Design review of the part built by this model. Coordinates are the model's own, in mm. Face numbers are marked on the shaded views. A direction names the side the tool comes from. Give positions to 0.01 mm unless a question says otherwise; leave off trailing zeros. Order: outer loops, then holes, each group sorted by start corner. A loop starts at its lowest first (then second) coordinate and runs counter-clockwise, first axis right, second up.
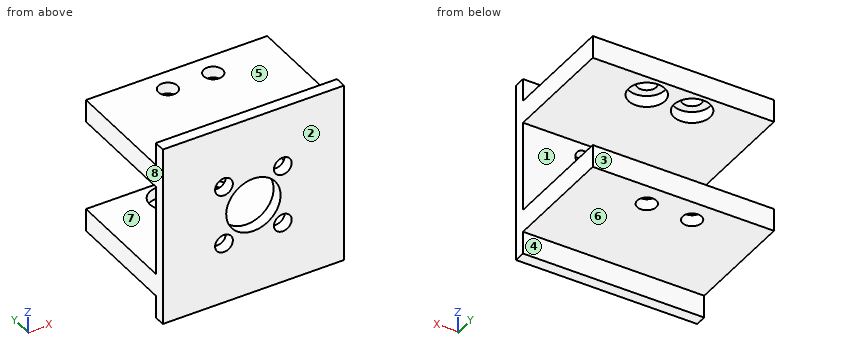
```python
from build123d import *

# Parameters (mm, degrees)
SKETCH1_W           = 50.8
SKETCH1_H           = 50.8
SKETCH1_R           = 2.4892
SKETCH1_R_2         = 7.62
BOSS_EXTRUDE1_DEPTH = 3.175
SKETCH2_W           = 50.8
SKETCH2_H           = 6.35
BOSS_EXTRUDE2_DEPTH = 31.75
CUT_EXTRUDE1_REACH  = 63.974
SKETCH3_R           = 2.667
SKETCH5_R           = 5.08
CUT_EXTRUDE2_DEPTH  = 3.175
CUT_EXTRUDE3_START  = -3.175
SKETCH6_R           = 5.08
CUT_EXTRUDE3_DEPTH  = 3.175


with BuildPart() as part:
    # Sketch1 → Boss-Extrude1 (new body)
    with BuildSketch(Plane(origin=(0, 0, 0), x_dir=(1, 0, 0), z_dir=(0, 1, 0))):
        Rectangle(SKETCH1_W, SKETCH1_H)
        with Locations(Location((-8.243875119, 8.243875119, 0), (0, 0, 270))):
            Circle(SKETCH1_R, mode=Mode.SUBTRACT)
        with Locations(Location((8.243875119, 8.243875119, 0), (0, 0, 270))):
            Circle(SKETCH1_R, mode=Mode.SUBTRACT)
        with Locations(Location((8.243875119, -8.243875119, 0), (0, 0, 270))):
            Circle(SKETCH1_R, mode=Mode.SUBTRACT)
        with Locations(Location((-8.243875119, -8.243875119, 0), (0, 0, 270))):
            Circle(SKETCH1_R, mode=Mode.SUBTRACT)
        with Locations(Location((0, 0, 0), (0, 0, 270))):
            Circle(SKETCH1_R_2, mode=Mode.SUBTRACT)
    extrude(amount=BOSS_EXTRUDE1_DEPTH)

    # Sketch2 → Boss-Extrude2 (add)
    with BuildSketch(Plane(origin=(0, 3.175, 0), x_dir=(1, 0, 0), z_dir=(0, 1, 0))):
        with Locations((0, 15.875)):
            Rectangle(SKETCH2_W, SKETCH2_H)
        with Locations((0, -15.875)):
            Rectangle(SKETCH2_W, SKETCH2_H)
    extrude(amount=BOSS_EXTRUDE2_DEPTH)

    # Cut-Extrude1: up to this face of the body (flat: up to its plane)
    cut_extrude1_end = Plane(part.part.faces().sort_by_distance((0, 19.05, 19.05))[0])
    # Sketch3 → Cut-Extrude1 (cut, up to the picked face)
    with BuildSketch(Plane(origin=(0, 0, -19.05), x_dir=(-1, 0, 0), z_dir=(0, 0, -1)), mode=Mode.PRIVATE) as cut_extrude1_sk1:
        with Locations((-6.35, 28.575)):
            Circle(SKETCH3_R)
    cut_extrude1_tool1 = split(extrude(cut_extrude1_sk1.sketch, amount=-CUT_EXTRUDE1_REACH, mode=Mode.PRIVATE), bisect_by=cut_extrude1_end, keep=Keep.BOTH, mode=Mode.PRIVATE)
    # Sketch3 → Cut-Extrude1 (cut, up to the picked face)
    with BuildSketch(Plane(origin=(0, 0, -19.05), x_dir=(-1, 0, 0), z_dir=(0, 0, -1)), mode=Mode.PRIVATE) as cut_extrude1_sk2:
        with Locations((6.35, 28.575)):
            Circle(SKETCH3_R)
    cut_extrude1_tool2 = split(extrude(cut_extrude1_sk2.sketch, amount=-CUT_EXTRUDE1_REACH, mode=Mode.PRIVATE), bisect_by=cut_extrude1_end, keep=Keep.BOTH, mode=Mode.PRIVATE)
    add(cut_extrude1_tool1.solids().sort_by(Axis((6.35, 28.575, -19.05), (0, 0, 1)))[0], mode=Mode.SUBTRACT)
    add(cut_extrude1_tool2.solids().sort_by(Axis((-6.35, 28.575, -19.05), (0, 0, 1)))[0], mode=Mode.SUBTRACT)

    # Sketch5 → Cut-Extrude2 (cut)
    with BuildSketch(Plane.XY.offset(-12.7)):
        with Locations((-6.35, 28.575)):
            Circle(SKETCH5_R)
        with Locations((6.35, 28.575)):
            Circle(SKETCH5_R)
    extrude(amount=-CUT_EXTRUDE2_DEPTH, mode=Mode.SUBTRACT)

    # Sketch6 → Cut-Extrude3 (cut)
    with BuildSketch(Plane(origin=(0, 0, 12.7), x_dir=(-1, 0, 0), z_dir=(0, 0, -1)).offset(CUT_EXTRUDE3_START)):
        with Locations(Location((-6.35, 28.575, 0), (0, 0, 180))):
            Circle(SKETCH6_R)
        with Locations(Location((6.35, 28.575, 0), (0, 0, 180))):
            Circle(SKETCH6_R)
    extrude(amount=CUT_EXTRUDE3_DEPTH, mode=Mode.SUBTRACT)


solid = part.part
```
1. Machinability: for the marked faces 1, 2, 3, 4 and 5, which of the approach directions +Z, -Z, +X, -X, +Y, -Y give a long, thin tool a straight path to every point of the face, cutting with its end or side? Answer none if there is none.
Recorded:
face 1: +X, -X, +Y
face 2: +Z, -Z, +X, -X, -Y
face 3: +Z, -Z, +X, -X, +Y
face 4: -Z, +X, -X, +Y
face 5: +Z, +X, -X, +Y
2. Take a section at A-A (y = 9.5). State the section outline as (x, z) points, then the cut area to 3 significant figures.
Recorded:
outline: (-25.4, -19.05) - (25.4, -19.05) - (25.4, -12.7) - (-25.4, -12.7) - close; (-25.4, 12.7) - (25.4, 12.7) - (25.4, 19.05) - (-25.4, 19.05) - close
area: 645 mm2
3. For line 1 along Z through (x, y) = (21, 16.5); line 2 along Y through (x, z) = (6.35, 17.45) (3 decimals); line 3 along Y through (x, z) = (6, -14) (3 decimals), list the stretches that pass through material, from the lowest coordinate up.
Recorded:
line 1: z = -19.05 to -12.7, 12.7 to 19.05
line 2: y = 0 to 25.908, 31.242 to 34.925
line 3: y = 0 to 23.507, 33.643 to 34.925
4. Take a section at D-D (x = -14.5). State the section outline as (y, z) points (3 decimals), then the cut area to 3 significant figures.
Recorded:
outline: (0, -25.4) - (3.175, -25.4) - (3.175, -19.05) - (34.925, -19.05) - (34.925, -12.7) - (3.175, -12.7) - (3.175, 12.7) - (34.925, 12.7) - (34.925, 19.05) - (3.175, 19.05) - (3.175, 25.4) - (0, 25.4) - close
area: 565 mm2
5. Take a section at C-C (z = 8.5). State the section outline as (x, y) points (3 decimals), then the cut area to 3 significant figures.
Recorded:
outline: (-25.4, 0) - (-10.72, 0) - (-10.72, 3.175) - (-25.4, 3.175) - close; (-5.768, 0) - (5.768, 0) - (5.768, 3.175) - (-5.768, 3.175) - close; (10.72, 0) - (25.4, 0) - (25.4, 3.175) - (10.72, 3.175) - close
area: 130 mm2
6. For pin 1 (5 mm diameter, centred on x = -4.5, z = -22.5, fed in from +Y) (3 decimals); pin 2 (3 mm diameter, centred on x = 6.35, y = 28.575, fed in from +Z) (3 decimals); pin 3 (8 mm diameter, centred on x = -5.5, y = 18.5, fed in from -Z); pin 4 (11 mm diameter, centred on x = -8.5, y = 27, fed in from +Z), all flat-tipped, find the tip position at first contact; note any pin that passes through.
Recorded:
pin 1: stops at y = 3.175
pin 2: passes through
pin 3: stops at z = -19.05
pin 4: stops at z = 19.05
7. Draft analysis for pull direction Z (two halves, no side actions). For the marked faces 6, 7 and 8, state which applies: pulls with the +Z half, pulls with the -Z half, needs draft (parallel to the pull), parting line crosses it, or undercut.
Recorded:
face 6: pulls with the -Z half
face 7: undercut
face 8: needs draft
8. Take a section at B-B (x = 0). State the section outline as (y, z) points (3 decimals), then the cut area to 3 significant figures.
Recorded:
outline: (0, -25.4) - (3.175, -25.4) - (3.175, -19.05) - (34.925, -19.05) - (34.925, -12.7) - (3.175, -12.7) - (3.175, -7.62) - (0, -7.62) - close; (0, 7.62) - (3.175, 7.62) - (3.175, 12.7) - (34.925, 12.7) - (34.925, 19.05) - (3.175, 19.05) - (3.175, 25.4) - (0, 25.4) - close
area: 516 mm2
